Verification items for the finished model (mm, model axes). Coordinates: 2 decimals unless noted, no trailing zeros. Order: outer loops, then holes, each group sorted by start corner. A loop starts at its lowest first (then second) coordinate and runs counter-clockwise, first axis right, second up. Notation, with made-up numbers: M -2,60.25 L 21,60.25 A19 ccw 21,66.25 Z; hole C -38.75,32 d4. An arc over 180 degrees is marked long. Return JSON: item names as keys, results as strings. Group by question number.
Q1. Thickness scan on probe 1 along Z at (x, y) = (-0.75, -3.5); probe 2 along Y at (x, z) = (-1.25, 2.25); probe 3 along X at (y, z) = (0.75, 1). Record the ranges inside material, lowest first.
Q2. Section check C-C, the plane z = 6. Enter the section's corners in (x, y), then the cut area to 3 significant figures.
Q3. Go/stop test with flat-tipped pins: pin 1 Ø1 at (x, z) = (3, 3) entering from -Y; pin 2 Ø3 at (x, z) = (-2, 3.5) entering from +Y. Record where each tip stops, or that it passes through.
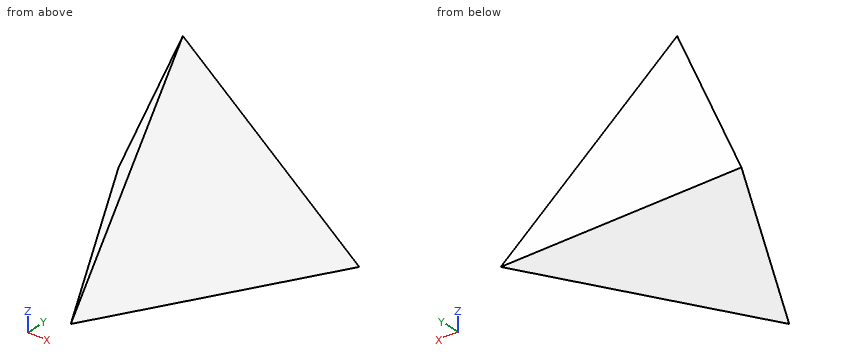
Solid Edge part; units mm, degrees
sketch "Sketch1" plane through (0, 0, 0) normal (0, 0, 1) x (1, 0, 0)
  line L0 (0, -5.7735) -> (5, 2.8868)
  line L1 (5, 2.8868) -> (-5, 2.8868)
  line L2 (-5, 2.8868) -> (0, -5.7735)
extrude "Protrusion1" add sketch "Sketch1" along normal up to vertex (8.165 mm away)
sketch "Sketch2" plane through (0, 0, 0) normal (1, 0, 0) x (0, 1, 0)
  line L0 (2.8868, 8.165) -> (0, 8.165)
  line L1 (0, 8.165) -> (2.8868, 0)
  line L2 (2.8868, 0) -> (2.8868, 8.165)
extrude "Cutout1" cut sketch "Sketch2" along normal mid plane 10
pattern_circular "Pattern1" count 3 over 360 about axis through (0, 0, 0) along (0, 0, 1) of "Cutout1"
Numbers:
{
 "1": {"probe 1": "z = 0 to 1.38", "probe 2": "y = -2.02 to 2.09", "probe 3": "x = -3.36 to 3.36"},
 "2": {"outline": "M -1.33,0.77 L 0,-1.53 L 1.33,0.77 Z", "area": "3.04 mm2"},
 "3": {"pin 1": "stops at y = 0.61", "pin 2": "stops at y = 2.18"}
}
